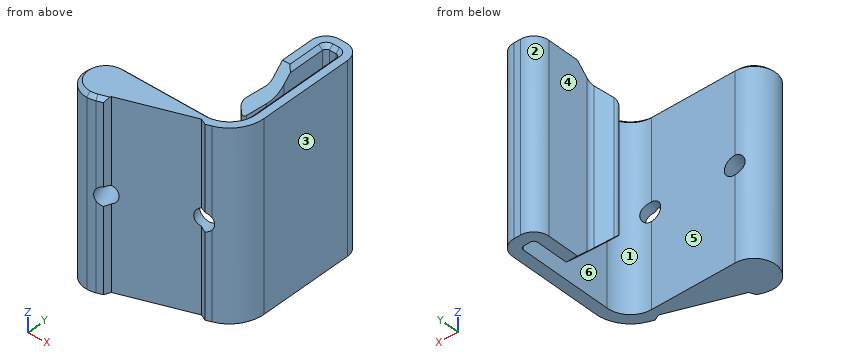
from build123d import *

# Parameters (mm, degrees)
BOSS_EXTRUDE1_DEPTH = 40
CUT_EXTRUDE2_DEPTH  = 53.049260875
SKETCH4_R           = 2
CUT_EXTRUDE3_DEPTH  = 10
CHAMFER2_SIZE       = 0.8
CUT_EXTRUDE1_DEPTH  = 54.113704366
FILLET2_R           = 0.8


with BuildPart() as part:
    # Sketch1 → Boss-Extrude1 (new body)
    with BuildSketch(Plane.XY):
        with BuildLine():
            Line((2.4, 0), (2.4, 9.2))
            ThreePointArc((2.4, 9.2), (2.634314575, 9.765685425), (3.2, 10))
            Line((3.2, 10), (4.6, 10))
            ThreePointArc((4.6, 10), (5.165685425, 9.765685425), (5.4, 9.2))
            Line((5.4, 9.2), (5.4, -10.8))
            ThreePointArc((5.4, -10.8), (3.935533906, -14.335533906), (0.4, -15.8))
            Line((0.4, -15.8), (-17.573004072, -15.8))
            ThreePointArc((-17.573004072, -15.8), (-22.12083665, -20.347832578), (-17.573004072, -24.895665156))
            ThreePointArc((-17.573004072, -24.895665156), (-16.704763183, -24.819703921), (-15.862903355, -24.59412826))
            Line((-15.862903355, -24.59412826), (2.930949061, -17.753725394))
            ThreePointArc((2.930949061, -17.753725394), (6.461725128, -15.044465629), (7.8, -10.8))
            Line((7.8, -10.8), (7.8, 9.2))
            ThreePointArc((7.8, 9.2), (6.8627417, 11.4627417), (4.6, 12.4))
            Line((4.6, 12.4), (3.2, 12.4))
            ThreePointArc((3.2, 12.4), (0.9372583, 11.4627417), (0, 9.2))
            Line((0, 9.2), (0, 0))
            ThreePointArc((0, 0), (-0.121792748, -0.612293492), (-0.46862915, -1.13137085))
            Line((-0.46862915, -1.13137085), (-3.297056275, -3.959797975))
            Line((-3.297056275, -3.959797975), (-1.6, -5.656854249))
            Line((-1.6, -5.656854249), (1.228427125, -2.828427125))
            ThreePointArc((1.228427125, -2.828427125), (2.09551813, -1.530733729), (2.4, 0))
        make_face()
    extrude(amount=BOSS_EXTRUDE1_DEPTH)

    # Sketch3 → Cut-Extrude2 (cut, through all)
    with BuildSketch(Plane.XY.offset(40)):
        Polygon((-14.090615102, -22.884890317), (0.474620521, -17.583578096), (1.756333285, -18.181250573), (-14.688287579, -24.166603081), align=None)
    extrude(amount=-CUT_EXTRUDE2_DEPTH, mode=Mode.SUBTRACT)

    # Sketch4 → Cut-Extrude3 (cut)
    with BuildSketch(Plane(origin=(6.048793264, -16.618922909, 0), x_dir=(0.939692620785907, 0.34202014332567265, 0), z_dir=(0.34202014332567265, -0.939692620785907, 0))):
        with Locations(Location((-4.901273833, 20, 0), (0, 0, 322.341537994))):
            Circle(SKETCH4_R)
        with Locations(Location((-21.734607166, 20, 0), (0, 0, 289.471220634))):
            Circle(SKETCH4_R)
    extrude(amount=-CUT_EXTRUDE3_DEPTH, mode=Mode.SUBTRACT)

    # Chamfer2
    chamfer2_edges = [part.edges().sort_by_distance(p)[0] for p in [
        (-0.185786438, -4.242640687, 40),
        (2.09551813, -1.530733729, 40),
        (2.4, 4.6, 40),
        (2.634314575, 9.765685425, 40),
        (3.9, 10, 40),
        (5.165685425, 9.765685425, 40),
        (5.4, -0.8, 40),
        (3.935533906, -14.335533906, 40),
        (-8.586502036, -15.8, 40),
        (-22.12083665, -20.347832578, 40),
        (-16.704763183, -24.819703921, 40),
        (-15.275595467, -24.380365671, 40),
    ]]
    chamfer(chamfer2_edges, length=CHAMFER2_SIZE)

    # Sketch2 → Cut-Extrude1 (cut, through all)
    with BuildSketch(Plane(origin=(2.4, 0, 0), x_dir=(0, 0, -1), z_dir=(1, 0, 0))):
        Polygon((-40, 2.343145751), (-32, -5.656854249), (-40, -5.656854249), align=None)
        Polygon((0, 2.343145751), (-8, -5.656854249), (0, -5.656854249), align=None)
    extrude(amount=-CUT_EXTRUDE1_DEPTH, mode=Mode.SUBTRACT)

    # Fillet2
    fillet2_edges = [part.edges().sort_by_distance(p)[0] for p in [
        (-1.6, -5.656854249, 20),
        (-3.297056275, -3.959797975, 20),
    ]]
    fillet(fillet2_edges, radius=FILLET2_R)


solid = part.part
Could you check a few things on this model? Use its own coordinates, in mm. Face numbers are marked on the shaded views. A direction names the side the tool comes from. Give positions to 0.01 mm unless a question says otherwise; leave off trailing zeros. Loops run counter-clockwise (first coordinate to the right, second up) from the corner with the lowest first, then second, coordinate; pieces in that order, holes last. Notation, with made-up numbers: M 13.25,49.5 L 53.25,49.5 A28 cw 53.25,72.5 Z; hole C 82.25,54.5 d2. An arc over 180 degrees is marked long. Answer as a JSON object with one key per item and string values.
Q1. Suppose I cut it at B-B, the plane z = 20.5. List the corners of the cut face in (x, y) for me.
Values found:
{"outline": "M -19.31,-16.15 A4.55 ccw -17.57,-24.9 A5 ccw -16.2,-24.7 Z; M -15.32,-15.8 L -12.9,-22.45 L -0.72,-18.02 L -1.53,-15.8 Z; M -2.73,-4.53 L -2.17,-5.09 A0.8 ccw -1.03,-5.09 L 1.23,-2.83 A4 ccw 2.4,0 L 2.4,9.2 A0.8 cw 3.2,10 L 4.6,10 A0.8 cw 5.4,9.2 L 5.4,-10.8 A5 cw 2.44,-15.37 L 3.26,-17.63 A7.4 ccw 7.8,-10.8 L 7.8,9.2 A3.2 ccw 4.6,12.4 L 3.2,12.4 A3.2 ccw 0,9.2 L 0,0 A1.6 cw -0.47,-1.13 L -2.73,-3.39 A0.8 ccw Z"}
Q2. Suppose I cut it at D-D, the plane x = -4. List the corners of the cut face in (y, z) for me, plus the area to 3 significant figures.
Values found:
{"outline": "M -19.21,0 L -15.8,0 L -15.8,39.2 L -16.6,40 L -19.21,40 Z", "area": "136 mm²"}
Q3. For the marked faces 4, 5 and 6, which set-ups out of +Z, -Z, +X, -X, +Y, -Y let a thin tool reach every point of the face, with its end or its side?
Values found:
{"face 4": "+Z, -Z, -X, +Y", "face 5": "+Z, -Z, -X", "face 6": "+Z, -Z"}
Q4. If we mould it in two halves opening along Y, with no side actions, what happens to the marked faces 1, 2 and 3? For each: pulls with the +Y half, pulls with the -Y half, needs draft (parallel to the pull), parting line crosses it, or undercut.
Values found:
{"face 1": "undercut", "face 2": "pulls with the +Y half", "face 3": "needs draft"}
Q5. For P1, Ø10, axis at y = 1.5, z = 19.5, coming from the -X side; P2, Ø8, axis at x = -3, z = 15.5, coming from the -Y side; P3, Ø1.5, axis at y = -13, z = 10, coming from the +X side, each with a flat end and sliding along its axis, tell me the tip position at first contact or that it passes through.
Values found:
{"P1": "stops at x = -2.82", "P2": "stops at y = -20.3", "P3": "stops at x = 7.66"}
Q6. Suppose I cut it at A-A, the plane y = 6. List the corners of the cut face in (x, z) for me, plus the area to 3 significant figures.
Values found:
{"outline": "M 0,0 L 2.4,0 L 2.4,39.2 L 1.6,40 L 0,40 Z; M 5.4,0 L 7.8,0 L 7.8,40 L 6.2,40 L 5.4,39.2 Z", "area": "191 mm²"}
Q7. If I drill on probe 1 along X at (y, z) = (2, 22); probe 2 along Y at (x, z) = (-16.25, 22.5); probe 3 along X at (y, z) = (-11, 26), over which ranges is the centre line in solid material (lowest first)? Write a range as [from, to].
Values found:
{"probe 1": "x = [0, 2.4], [5.4, 7.8]", "probe 2": "y = [-24.72, -15.8]", "probe 3": "x = [5.4, 7.8]"}
Q8. Suppose I cut it at C-C, the plane z = 28. List the corners of the cut face in (x, y) for me, plus the area to 3 significant figures.
Values found:
{"outline": "M -17.57,-24.9 A5 ccw -15.86,-24.59 L -14.69,-24.17 L -14.09,-22.88 L 0.47,-17.58 L 1.76,-18.18 L 2.93,-17.75 A7.4 ccw 7.8,-10.8 L 7.8,9.2 A3.2 ccw 4.6,12.4 L 3.2,12.4 A3.2 ccw 0,9.2 L 0,0 A1.6 cw -0.47,-1.13 L -2.73,-3.39 A0.8 ccw -2.73,-4.53 L -2.17,-5.09 A0.8 ccw -1.03,-5.09 L 1.23,-2.83 A4 ccw 2.4,0 L 2.4,9.2 A0.8 cw 3.2,10 L 4.6,10 A0.8 cw 5.4,9.2 L 5.4,-10.8 A5 cw 0.4,-15.8 L -17.57,-15.8 A4.55 ccw Z", "area": "253 mm²"}
